Job drawing, mm, ordinate dimensions from the low corner. One solid piece. A direction names the side the tool comes from. Give positions to 0.01 mm unless a question says otherwise; leave off trailing zeros. Write each loop counter-clockwise with the first axis right and the second up, starting at its lowest first coordinate (ties: lowest second). Pieces come first, ordered by that corner, then holes. Notation, with made-up numbers: M -21,7 L 24,7 A14 ccw 24,32 Z; hole C 28,15 d1. An arc over 180 degrees is marked long. Use a Markdown table: item, result.
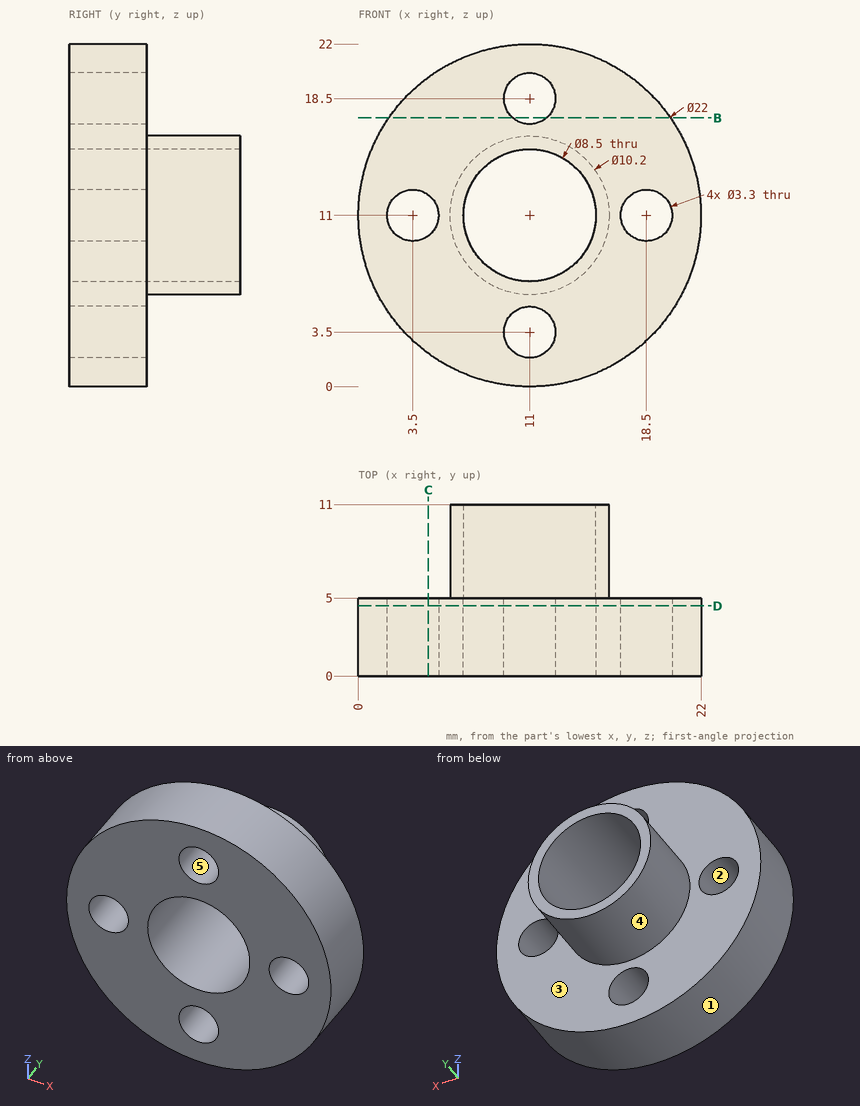
1. Drill centre lines: L1, parallel to Z at x = 11, y = 2.95; L2, parallel to X at y = 7.5, z = 11; L3, parallel to Y at x = 15.5, z = 7.5. Where is each one in solid material? Low to high.
Findings below:
| item | result |
|---|---|
| L1 | 0 to 1.85, 5.15 to 6.75, 15.25 to 16.85, 20.15 to 22 |
| L2 | 5.9 to 6.75, 15.25 to 16.1 |
| L3 | 0 to 5 |
2. Cut at C-C, the plane x = 4.5. Give the cut face in (y, z), then the cut area to 3 significant figures.
Findings below:
| item | result |
|---|---|
| outline | M 0,2.13 L 5,2.13 L 5,9.69 L 0,9.69 Z; M 0,12.31 L 5,12.31 L 5,19.87 L 0,19.87 Z |
| area | 75.6 mm2 |
3. Cut at B-B, the plane z = 17.25. Give the cut face in (x, y).
Findings below:
| item | result |
|---|---|
| outline | M 1.95,0 L 9.92,0 L 9.92,5 L 1.95,5 Z; M 12.08,0 L 20.05,0 L 20.05,5 L 12.08,5 Z |
4. Drop flat-ended pins along their axis: P1, Ø3, axis at y = 1.5, z = 5.5, coming from the -X side; P2, Ø5, axis at x = 17, z = 4, coming from the +Y side; P3, Ø2, axis at y = 7.5, z = 12.5, coming from the +X side. Give the stop position or say it passes through.
Findings below:
| item | result |
|---|---|
| P1 | x = 0.75 |
| P2 | y = 5 |
| P3 | x = 16.08 |
5. Cut at D-D, the plane y = 4.5. Give the cut face in (x, z), then the cut area to 3 significant figures.
Findings below:
| item | result |
|---|---|
| outline | C 11,11 d22; hole C 3.5,11 d3.3; hole C 11,11 d8.5; hole C 11,3.5 d3.3; hole C 11,18.5 d3.3; hole C 18.5,11 d3.3 |
| area | 289 mm2 |
6. Tool access for the marked faces 4 and 5: list every direction of +Z, -Z, +X, -X, +Y, -Y with a clear straight run to the whole face (end or side of a thin tool).
Findings below:
| item | result |
|---|---|
| face 4 | +Y |
| face 5 | +Y, -Y |
7. Two-plate mould, pull along Z, no slides. Class the marked faces 1, 2 and 3: released by +Z, released by -Z, zero draft, split by the parting line, or undercut.
Findings below:
| item | result |
|---|---|
| face 1 | split by the parting line |
| face 2 | undercut |
| face 3 | zero draft |
